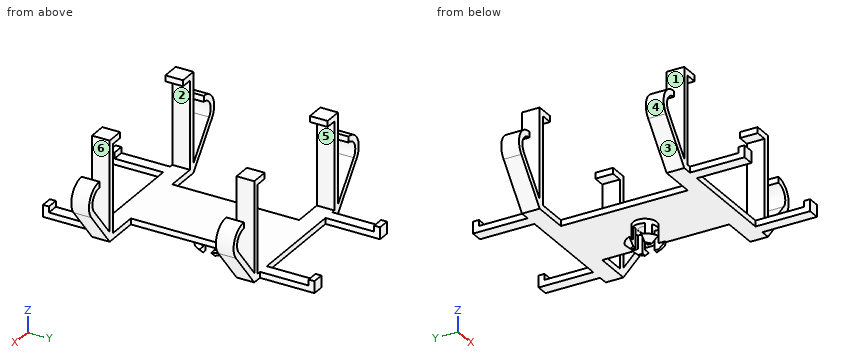
```python
from build123d import *

# Parameters (mm, degrees)
F3_DEPTH  = 27.5
F5_DEPTH  = 27.5
F4_W      = 15.75
F4_H      = 43
F4_W_2    = 12.25
F6_DEPTH  = 33.751
F8_DEPTH  = 21
F10_DEPTH = 33.751
F11_W     = 2
F11_H     = 6.5
F12_DEPTH = 10
F13_W     = 2
F13_H     = 6.5
F14_DEPTH = 12.5


with BuildPart() as f1:
    # F0 (on Front) → F1 (revolve)
    with BuildSketch(Plane.XZ):
        Polygon((2, -16.875), (0, -16.875), (0, -18.3531418443), (2, -18.3531418443), (2, -24.875), (4, -24.875), (6, -22.875), (4, -22.875), (4, -16.875), align=None)
    revolve(axis=Axis((0, 0, -17.6140709221), (0, 0, 1)))

    # F0 (on Front) → F3 (join, symmetric)
    with BuildSketch(Plane.XZ):
        Polygon((-22.25, -14.875), (-22.25, 14.875), (-18.25, 14.875), (-18.25, 16.875), (-24.25, 16.875), (-24.25, -16.875), (0, -16.875), (2, -16.875), (4, -16.875), (24.25, -16.875), (24.25, 16.875), (18.25, 16.875), (18.25, 14.875), (22.25, 14.875), (22.25, -14.875), align=None)
    extrude(amount=F3_DEPTH, both=True)

    # F2 (on Front) → F5 (join, symmetric)
    with BuildSketch(Plane.XZ):
        with BuildLine():
            ThreePointArc((30.25, 4), (33.8625360184, 1.7174351563), (33.3521481806, -2.525208242))
            Line((33.3521481806, -2.525208242), (24.25, -13.7069444444))
            Line((24.25, -13.7069444444), (24.25, -16.875))
            Line((24.25, -16.875), (34.9032222709, -3.787812363))
            ThreePointArc((34.9032222709, -3.787812363), (35.6688040276, 2.5761527344), (30.25, 6))
            Line((30.25, 6), (30.25, 4))
        make_face()
        with BuildLine():
            ThreePointArc((-30.25, 6), (-35.6688040276, 2.5761527344), (-34.9032222709, -3.787812363))
            Line((-34.9032222709, -3.787812363), (-24.25, -16.875))
            Line((-24.25, -16.875), (-24.25, -13.7069444444))
            Line((-24.25, -13.7069444444), (-33.3521481806, -2.525208242))
            ThreePointArc((-33.3521481806, -2.525208242), (-33.8625360184, 1.7174351563), (-30.25, 4))
            Line((-30.25, 4), (-30.25, 6))
        make_face()
    extrude(amount=F5_DEPTH, both=True)

    # F4 (on face) → F6 (cut, through all)
    with BuildSketch(Plane(origin=(0, 0, -16.875), x_dir=(1, 0, 0), z_dir=(0, 0, -1))):
        with Locations((-32.125, 0)):
            Rectangle(F4_W, F4_H)
        with Locations((-18.125, 0)):
            Rectangle(F4_W_2, F4_H)
        with Locations((18.125, 0)):
            Rectangle(F4_W_2, F4_H)
        with Locations((32.125, 0)):
            Rectangle(F4_W, F4_H)
    extrude(amount=-F6_DEPTH, mode=Mode.SUBTRACT)

    # F7 (on Right) → F8 (join, symmetric)
    with BuildSketch(Plane.YZ):
        Polygon((-46, -16.875), (-27.5, -16.875), (-27.5, -14.875), (-44, -14.875), (-44, -12.875), (-46, -12.875), align=None)
        Polygon((46, -16.875), (46, -12.875), (44, -12.875), (44, -14.875), (27.5, -14.875), (27.5, -16.875), align=None)
    extrude(amount=F8_DEPTH, both=True)

    # F9 (on face) → F10 (cut, through all)
    with BuildSketch(Plane(origin=(0, 0, -16.875), x_dir=(1, 0, 0), z_dir=(0, 0, -1))):
        Polygon((17, 46), (-17, 46), (-17, 27.5), (0, 27.5), (17, 27.5), align=None)
        Polygon((-17, -27.5), (-17, -46), (17, -46), (17, -27.5), (0, -27.5), align=None)
    extrude(amount=-F10_DEPTH, mode=Mode.SUBTRACT)

    # F11 (on Front) → F12 (cut, symmetric)
    with BuildSketch(Plane.XZ):
        with Locations((1, -21.6578255147)):
            Rectangle(F11_W, F11_H)
        with Locations((-1, -21.6578255147)):
            Rectangle(F11_W, F11_H)
    extrude(amount=F12_DEPTH, both=True, mode=Mode.SUBTRACT)

    # F13 (on Right) → F14 (cut, symmetric)
    with BuildSketch(Plane.YZ):
        with Locations((1, -21.625)):
            Rectangle(F13_W, F13_H)
        with Locations((-1, -21.625)):
            Rectangle(F13_W, F13_H)
    extrude(amount=F14_DEPTH, both=True, mode=Mode.SUBTRACT)


solid = f1.part
```
Could you check a few things on this model? Use its own coordinates, in mm. Face numbers are marked on the shaded views. A direction names the side the tool comes from. Round coordinates to 2 decimals unless told otherwise and drop trailing zeros. Loops run counter-clockwise (first coordinate to the right, second up) from the corner with the lowest first, then second, coordinate; pieces in that order, holes last. Notation, with made-up numbers: M 28,11 L 52,11 A28 ccw 52,49 Z; hole C 10.5,32.5 d8. An arc over 180 degrees is marked long. Put each result on its own line as item: value.
Q1. Thinking about a two-plate mould opening in Z: for the marked faces 1, 2 and 3, which applies, released by +Z, released by -Z, zero draft, split by the parting line, or undercut?
Check result:
face 1: zero draft
face 2: undercut
face 3: released by -Z
Q2. For pin 1 (3 mm diameter, centred on y = 40, z = -14, fed in from +X); pin 2 (1 mm diameter, centred on y = 0, z = -15.5, fed in from +X); pin 3 (3 mm diameter, centred on x = 21.5, y = -34, fed in from -Z) (3 decimals), each with a flat end and sliding along its axis, tell me the tip position at first contact or that it passes through.
Check result:
pin 1: x = 21
pin 2: x = 12
pin 3: z = -16.875
Q3. Imagine slicing it at C-C (y = -30.5). Write out the boundary of the cut face in (x, z) (3 decimals).
Check result:
outline: M -21,-16.875 L -17,-16.875 L -17,-14.875 L -21,-14.875 Z; M 17,-16.875 L 21,-16.875 L 21,-14.875 L 17,-14.875 Z
Q4. Imagine slicing it at B-B (z = 13). Write out the boundary of the cut face in (x, y), then the cut area to 3 significant figures.
Check result:
outline: M -24.25,-27.5 L -22.25,-27.5 L -22.25,-21.5 L -24.25,-21.5 Z; M -24.25,21.5 L -22.25,21.5 L -22.25,27.5 L -24.25,27.5 Z; M 22.25,-27.5 L 24.25,-27.5 L 24.25,-21.5 L 22.25,-21.5 Z; M 22.25,21.5 L 24.25,21.5 L 24.25,27.5 L 22.25,27.5 Z
area: 48.0 mm2
Q5. Imagine slicing it at D-D (y = 0). Write out the boundary of the cut face in (x, z) (3 decimals).
Check result:
outline: M -12,-16.875 L -4,-16.875 L -4,-18.375 L -2,-18.375 L -2,-18.353 L 2,-18.353 L 2,-18.375 L 4,-18.375 L 4,-16.875 L 12,-16.875 L 12,-14.875 L -12,-14.875 Z
Q6. I need wall thicknesses on probe 1 along Z at (x, y) = (20, -24) (3 decimals); probe 2 along Y at (x, z) = (31, 4); probe 3 along X at (y, z) = (0, -18). Which ranges of each line are inside material? Lowest first, please.
Check result:
probe 1: -16.875 to -14.875, 14.875 to 16.875
probe 2: -27.5 to -21.5, 21.5 to 27.5
probe 3: -4 to 4
Q7. On a 3-axis mill with a long thin cutter (end or side, diameter ignored), from which of +Z, -Z, +X, -X, +Y, -Y can I reach the whole of each face in a straight line? I mean the marked faces 4, 5 and 6. Say none if no direction works.
Check result:
face 4: -X, +Y, -Y
face 5: +Y, -Y
face 6: +Z, +Y, -Y
Q8. Imagine slicing it at A-A (x = -13.5). Write out the boundary of the cut face in (y, z) (3 decimals).
Check result:
outline: M -27.5,-16.875 L -21.5,-16.875 L -21.5,-14.875 L -27.5,-14.875 Z; M 21.5,-16.875 L 27.5,-16.875 L 27.5,-14.875 L 21.5,-14.875 Z
